Can you work these out from the model? Positions are in its coordinate system, mm. A direction names the side the tool comes from. Round coordinates to 2 decimals unless told otherwise and drop trailing zeros. Loops run counter-clockwise (first coordinate to the right, second up) from the corner with the lowest first, then second, coordinate; pieces in that order, holes last.
from build123d import *

# Parameters (mm, degrees)
SKETCH1_R                = 39.2
SKETCH1_R_2              = 2.5527
BOSS_EXTRUDE1_DEPTH      = 2.032
BOSS_EXTRUDE5_DEPTH      = 2.032
FILLET2_R                = 1.016
CIRPATTERN2_COUNT        = 5
FILLET2_OF_CIRPATTERN2_R = 1.016


with BuildPart() as part:
    # Sketch1 → Boss-Extrude1 (new body)
    with BuildSketch(Plane.XY):
        Circle(SKETCH1_R)
        with BuildLine():
            ThreePointArc((24.820271985, 19.799409047), (25.601853519, 16.808343049), (23.907855902, 14.222280874))
            ThreePointArc((23.907855902, 14.222280874), (21.312007949, 6.924691149), (27.701508676, 2.546618187))
            ThreePointArc((27.701508676, 2.546618187), (30.592030744, 1.450156756), (31.717822482, -1.429068567))
            ThreePointArc((31.717822482, -1.429068567), (30.196044392, -9.811289571), (26.500242841, -17.487127533))
            ThreePointArc((26.500242841, -17.487127533), (23.89709201, -19.154745969), (20.914126675, -18.342795657))
            ThreePointArc((20.914126675, -18.342795657), (13.171545281, -18.12907679), (10.982214772, -25.558752039))
            ThreePointArc((10.982214772, -25.558752039), (10.832638425, -28.646627104), (8.442221199, -30.607048228))
            ThreePointArc((8.442221199, -30.607048228), (0, -31.75), (-8.442221199, -30.607048228))
            ThreePointArc((-8.442221199, -30.607048228), (-10.832638425, -28.646627104), (-10.982214772, -25.558752039))
            ThreePointArc((-10.982214772, -25.558752039), (-13.171545281, -18.12907679), (-20.914126675, -18.342795657))
            ThreePointArc((-20.914126675, -18.342795657), (-23.89709201, -19.154745969), (-26.500242841, -17.487127533))
            ThreePointArc((-26.500242841, -17.487127533), (-30.196044392, -9.811289571), (-31.717822482, -1.429068567))
            ThreePointArc((-31.717822482, -1.429068567), (-30.592030744, 1.450156756), (-27.701508676, 2.546618187))
            ThreePointArc((-27.701508676, 2.546618187), (-21.312007949, 6.924691149), (-23.907855902, 14.222280874))
            ThreePointArc((-23.907855902, 14.222280874), (-25.601853519, 16.808343049), (-24.820271985, 19.799409047))
            ThreePointArc((-24.820271985, 19.799409047), (-18.66218176, 25.686289571), (-11.160471144, 29.723835281))
            ThreePointArc((-11.160471144, 29.723835281), (-8.07427636, 29.542873268), (-6.138259129, 27.132648635))
            ThreePointArc((-6.138259129, 27.132648635), (0, 22.408771281), (6.138259129, 27.132648635))
            ThreePointArc((6.138259129, 27.132648635), (8.07427636, 29.542873268), (11.160471144, 29.723835281))
            ThreePointArc((11.160471144, 29.723835281), (18.66218176, 25.686289571), (24.820271985, 19.799409047))
        make_face(mode=Mode.SUBTRACT)
        with Locations((27.351216828, 8.886949063)):
            Circle(SKETCH1_R_2, mode=Mode.SUBTRACT)
        with Locations((0, 28.758771281)):
            Circle(SKETCH1_R_2, mode=Mode.SUBTRACT)
        with Locations((16.903981633, -23.266334704)):
            Circle(SKETCH1_R_2, mode=Mode.SUBTRACT)
        with Locations((-27.351216828, 8.886949063)):
            Circle(SKETCH1_R_2, mode=Mode.SUBTRACT)
        with Locations((-16.903981633, -23.266334704)):
            Circle(SKETCH1_R_2, mode=Mode.SUBTRACT)
    extrude(amount=BOSS_EXTRUDE1_DEPTH)

    # Sketch1<5> → Boss-Extrude5 (add)
    with BuildSketch(Plane.XY):
        with BuildLine():
            Line((-11.938, 43.595001502), (-9.536371101, 38.022330626))
            ThreePointArc((-9.536371101, 38.022330626), (-5.343297764, 38.83412377), (-1.086796161, 39.184931723))
            ThreePointArc((-1.086796161, 39.184931723), (-2.244635615, 39.285819975), (-3.349242804, 39.647225009))
            Line((-3.349242804, 39.647225009), (-11.938, 43.595001502))
        make_face()
        with BuildLine():
            ThreePointArc((3.349242804, 39.647225009), (2.244635615, 39.285819975), (1.086796161, 39.184931723))
            ThreePointArc((1.086796161, 39.184931723), (5.343297764, 38.83412377), (9.536371101, 38.022330626))
            Line((9.536371101, 38.022330626), (11.938, 43.595001502))
            Line((11.938, 43.595001502), (3.349242804, 39.647225009))
        make_face()
    boss_extrude5 = extrude(amount=BOSS_EXTRUDE5_DEPTH)

    # Fillet2
    fillet2_edges = [part.edges().sort_by_distance(p)[0] for p in [
        (-9.536371101, 38.022330626, 1.016),
        (9.536371101, 38.022330626, 1.016),
    ]]
    fillet(fillet2_edges, radius=FILLET2_R)

    # CirPattern2: Boss-Extrude5 ×5 about axis
    cirpattern2_axis = Axis((0, 0, 0), (0, 0, 1))
    for i in range(1, CIRPATTERN2_COUNT):
        add(boss_extrude5.rotate(cirpattern2_axis, i * 360 / CIRPATTERN2_COUNT))

    # Fillet2 of CirPattern2
    fillet2_of_cirpattern2_edges = [part.edges().sort_by_distance(p)[0] for p in [
        (-39.108286041, 2.679918452, 1.016),
        (-33.214484572, 20.819174207, 1.016),
        (-14.633878914, -36.366049936, 1.016),
        (-30.064051485, -25.155373348, 1.016),
        (30.064051485, -25.155373348, 1.016),
        (14.633878914, -36.366049936, 1.016),
        (33.214484572, 20.819174207, 1.016),
        (39.108286041, 2.679918452, 1.016),
    ]]
    fillet(fillet2_of_cirpattern2_edges, radius=FILLET2_OF_CIRPATTERN2_R)


solid = part.part
(1) Will this pin go through, and if not, where does the flat tip stop? P1, Ø4, axis at x = -16.9, y = -23.27, coming from the -Z side.
Worked answers:
P1: passes through
(2) If we mould it in two halves opening along X, with no side actions, what happens to faces 6 (the cylindrical face through (19.262, -24.244, 1.002)), 7 (the flat face through (42.681, 2.348, 1.002)), 8 (the cylindrical face through (24.89, -30.47, 1)), 9 (the flat face through (-18.31, -38.11, 1))? For each: released by +X, released by -X, zero draft, split by the parting line, or undercut.
Worked answers:
face 6: undercut
face 7: undercut
face 8: released by +X
face 9: released by -X
(3) If we section it at C-C, the plane y = 5: List the corners of the cut face in (x, z) for me.
Worked answers:
outline: (-42.49, 0) - (-22.33, 0) - (-22.33, 2.03) - (-42.49, 2.03) - close; (22.33, 0) - (42.49, 0) - (42.49, 2.03) - (22.33, 2.03) - close
(4) If we section it at D-D, the plane z = 0.85: State how many separate pieces and enclosed holes the cut face has, then the cut area to 3 significant figures.
Worked answers:
separate pieces: 1
enclosed holes: 6
area: 2,310 mm2
(5) If I drill on line 1 (X direction, y = 25, z = 0.85); line 2 (X direction, y = -24, z = 0.4); line 3 (Y direction, x = 24, z = 1.9), over which ranges is the centre line in solid material (lowest first)?
Worked answers:
line 1: x = -30.19 to -19.57, -5.12 to 5.12, 19.57 to 30.19
line 2: x = -30.99 to -19.35, -14.46 to -10.6, 10.6 to 14.46, 19.35 to 30.99
line 3: y = -31 to -19.14, 3.49 to 14.28, 20.79 to 30.99
(6) For faces 1 (the flat face through (15.422, -39.867, 1.002)), 2 (the cylindrical face through (37.286, 12.099, 1.002)), 3 (the cylindrical face through (-10.81, -28.69, 1)), 4 (the flat face through (-7.6, 41.6, 1)), 5 (the flat face through (-10.984, 41.38, 1.002)), which set-ups out of +Z, -Z, +X, -X, +Y, -Y let a thin tool reach every point of the face, with its end or its side?
Worked answers:
face 1: +Z, -Z, -Y
face 2: +Z, -Z, +X
face 3: +Z, -Z
face 4: +Z, -Z, +Y
face 5: +Z, -Z, -X
(7) If we section it at B-B, the plane y = -8: List the corners of the cut face in (x, z) for me (3 decimals).
Worked answers:
outline: (-38.375, 0) - (-30.726, 0) - (-30.726, 2.032) - (-38.375, 2.032) - close; (30.726, 0) - (38.375, 0) - (38.375, 2.032) - (30.726, 2.032) - close
(8) If we section it at A-A, the plane x = 0: List the corners of the cut face in (y, z) for me, then the cut area to 3 significant figures.
Worked answers:
outline: (-39.2, 0) - (-31.75, 0) - (-31.75, 2.03) - (-39.2, 2.03) - close; (22.41, 0) - (26.21, 0) - (26.21, 2.03) - (22.41, 2.03) - close; (31.31, 0) - (39.2, 0) - (39.2, 2.03) - (31.31, 2.03) - close
area: 38.9 mm2
